Design review of the part shown in the three views and the two pictorial views. Dimensions are in mm from the part's minimum x, y and z. Coordinates: 2 decimals unless noted, no trailing zeros. Loops run counter-clockwise (first coordinate to the right, second up) from the corner with the lowest first, then second, coordinate; pieces in that order, holes last. Notation, with made-up numbers: (58, 45.5) -> (66, 45.5) arc R20 ccw to (66, 73.5) -> close; hole circle Ø7 at (83.25, 68). An arc over 180 degrees is marked (long way). One line per item, written item: value. Start each with the question number.
1. Draft analysis for pull direction X (two halves, no side actions). For the marked faces 1, 2 and 3, state which applies: pulls with the +X half, pulls with the -X half, needs draft (parallel to the pull), parting line crosses it, or undercut.
2. Insertion check: pin 1 (3 mm diameter, centred on y = 20.5, z = 51.5, fed in from +X); pin 2 (3 mm diameter, centred on y = 6, z = 33, fed in from +X); pin 3 (1.7 mm diameter, centred on y = 24, z = 101, fed in from +X). Each pin has a flat end and moves straight along its axis. Give the tip position at first contact, or say it passes through.
3. Add section B-B on y = 16.25. Write out the cut boundary in (x, z), plus the area to 3 significant figures.
4. For probe 1 along Z at (x, y) = (74.5, 17); probe 2 along Y at (x, z) = (78.5, 98); probe 3 along Z at (x, y) = (78, 1.75) (1 decimal), list the stretches that pass through material, from the lowest coordinate up.
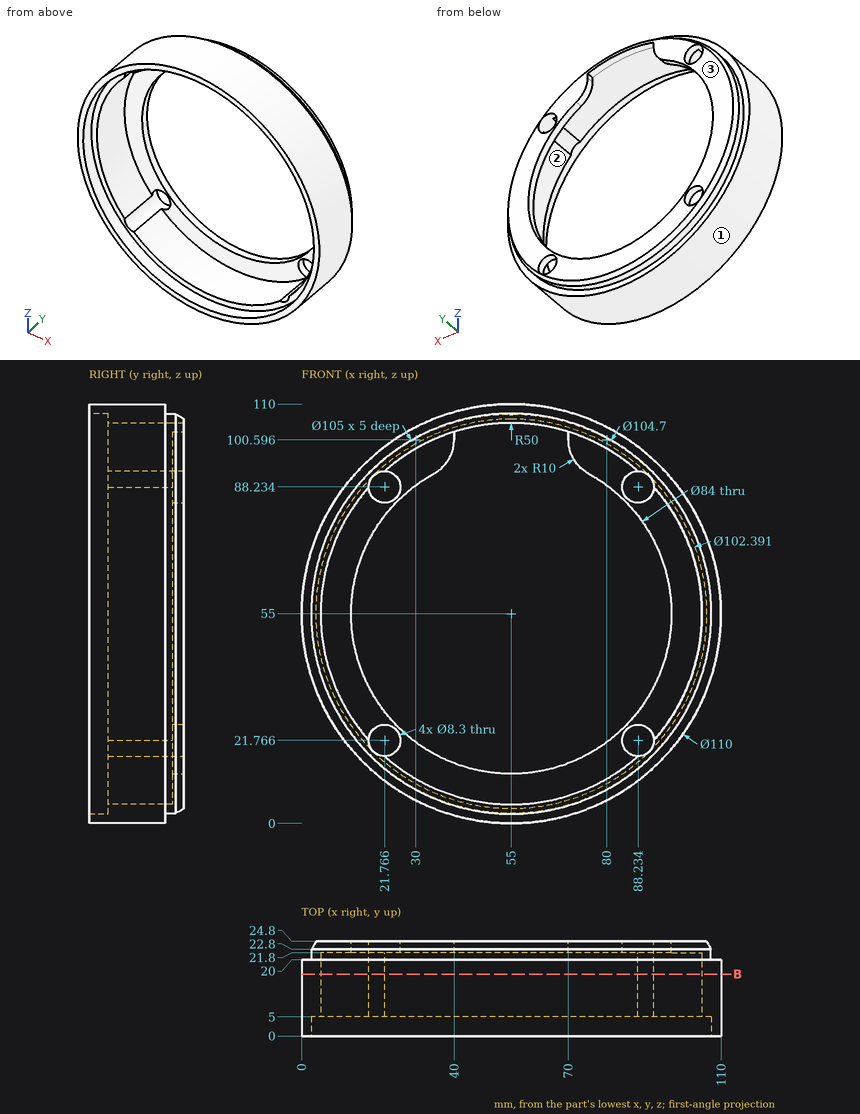
Worked answers:
1. face 1: parting line crosses it
1. face 2: undercut
1. face 3: needs draft
2. pin 1: stops at x = 109.96
2. pin 2: stops at x = 106.04
2. pin 3: stops at x = 80.4
3. outline: circle Ø110 at (55, 55); hole (17.62, 21.8) arc R4.15 ccw to (21.8, 17.62) arc R50 ccw to (88.2, 17.62) arc R4.15 ccw to (92.38, 21.8) arc R50 ccw to (92.38, 88.2) arc R4.15 ccw to (88.2, 92.38) arc R50 ccw to (21.8, 92.38) arc R4.15 ccw to (17.62, 88.2) arc R50 ccw to start
3. area: 1,630 mm²
4. probe 1: z = 3.57 to 8.96, 101.04 to 106.43
4. probe 2: y = 21.8 to 24.8
4. probe 3: z = 5 to 7.8, 102.2 to 105
